from build123d import *

# Parameters (mm, degrees)
BOSS_EXTRUDE1_DEPTH = 15
BOSS_EXTRUDE2_DEPTH = 4
FILLET1_R           = 2


with BuildPart() as part:
    # Sketch1 → Boss-Extrude1 (new body, symmetric)
    with BuildSketch(Plane(origin=(0, 0, 0), x_dir=(0, 0, -1), z_dir=(1, 0, 0))):
        Polygon((0, -12.5), (0, 12.5), (30, 12.5), (30, 8.5), (4, 8.5), (4, -12.5), align=None)
    extrude(amount=BOSS_EXTRUDE1_DEPTH, both=True)

    # Sketch2 → Boss-Extrude2 (add)
    with BuildSketch(Plane(origin=(15, 0, 0), x_dir=(0, 0, -1), z_dir=(1, 0, 0))):
        Polygon((30, 8.5), (4, -12.5), (4, 8.5), align=None)
    boss_extrude2 = extrude(amount=-BOSS_EXTRUDE2_DEPTH)

    # Mirror1: Boss-Extrude2 across plane
    add(boss_extrude2.mirror(Plane(origin=(0, 0, 0), x_dir=(0, 0, 1), z_dir=(1, 0, 0))))

    # Fillet1
    fillet1_edges = [part.edges().sort_by_distance(p)[0] for p in [
        (15, -12.5, -2),
        (15, 10.5, -30),
        (-15, -12.5, -2),
        (-15, 10.5, -30),
    ]]
    fillet(fillet1_edges, radius=FILLET1_R)


solid = part.part
Source: CAD feature listing. Evaluate the final solid. Frame: model axes, mm. A direction names the side the tool comes from. Give positions to 0.01 mm unless a question says otherwise; leave off trailing zeros. Order: outer loops, then holes, each group sorted by start corner. A loop starts at its lowest first (then second) coordinate and runs counter-clockwise, first axis right, second up. Notation, with made-up numbers: (-21.75, -15.75) -> (24.25, -15.75) arc R22 cw to (24.25, 8.25) -> close; hole circle Ø3 at (26.25, 10.25). An arc over 180 degrees is marked (long way). Use a Markdown table: item, result.
1) Ray query, line 1 along X through (y, z) = (7.5, -8.25); line 2 along Y through (x, z) = (0.75, -6.75); line 3 along Z through (x, y) = (1.75, 1.25). Return the intervals inside material, ascending. Write a range as [from, to].
Answer list:
| item | result |
|---|---|
| line 1 | [-15, -11], [11, 15] |
| line 2 | [8.5, 12.5] |
| line 3 | [-4, 0] |
2) Reachability of faces 1 (the flat face through (-11, 3, -11)), 2 (the flat face through (0, 0, 0)) from +Z, -Z, +X, -X, +Y, -Y: full face, straight path, thin tool, end or side. Return the list, or none.
Answer list:
| item | result |
|---|---|
| face 1 | -Z, -Y |
| face 2 | +Z, +X, -X, +Y, -Y |
3) Section query B-B, the plane z = -16.5. Return the cut outline in (x, y), then the cut area to 3 significant figures.
Answer list:
| item | result |
|---|---|
| outline | (-15, -2.4) -> (-11, -2.4) -> (-11, 8.5) -> (11, 8.5) -> (11, -2.4) -> (15, -2.4) -> (15, 12.5) -> (-15, 12.5) -> close |
| area | 207 mm² |
4) Section query C-C, the plane x = -7.5. Return the cut outline in (y, z).
Answer list:
| item | result |
|---|---|
| outline | (-12.5, -4) -> (8.5, -4) -> (8.5, -30) -> (12.5, -30) -> (12.5, 0) -> (-12.5, 0) -> close |
5) Section query A-A, the plane y = -9.5. Return the cut outline in (x, z), then the cut area to 3 significant figures.
Answer list:
| item | result |
|---|---|
| outline | (-15, -7.71) -> (-11, -7.71) -> (-11, -4) -> (11, -4) -> (11, -7.71) -> (15, -7.71) -> (15, 0) -> (-15, 0) -> close |
| area | 150 mm² |
6) Mould query, pull axis X, two halves, no side actions, for faces 3 (the flat face through (0, -12.5, -2)), 4 (the flat face through (0, 8.5, -17)), 5 (the cylindrical face through (-14.4, 10.28, -29.43)). Classes: +X half, -X half, draft (parallel to the pull), parting line (faces both ways), or undercut.
Answer list:
| item | result |
|---|---|
| face 3 | draft |
| face 4 | undercut |
| face 5 | -X half |
7) Section query D-D, the plane x = 11.5. Return the cut outline in (y, z), then the cut area to 3 significant figures.
Answer list:
| item | result |
|---|---|
| outline | (-12.5, -4) -> (8.5, -30) -> (12.5, -30) -> (12.5, 0) -> (-12.5, 0) -> close |
| area | 477 mm² |
8) Contact query for flat-ended pins moving along their axis: P1, Ø8, axis at x = -5.5, y = -5.5, coming from the -Z side; P2, Ø5, axis at x = -11, y = -8, coming from the -Z side; P3, Ø8, axis at x = -10, y = 8.5, coming from the +Z side. Output: stop coordinate, or through.
Answer list:
| item | result |
|---|---|
| P1 | z = -4 |
| P2 | z = -12.67 |
| P3 | z = 0 |
